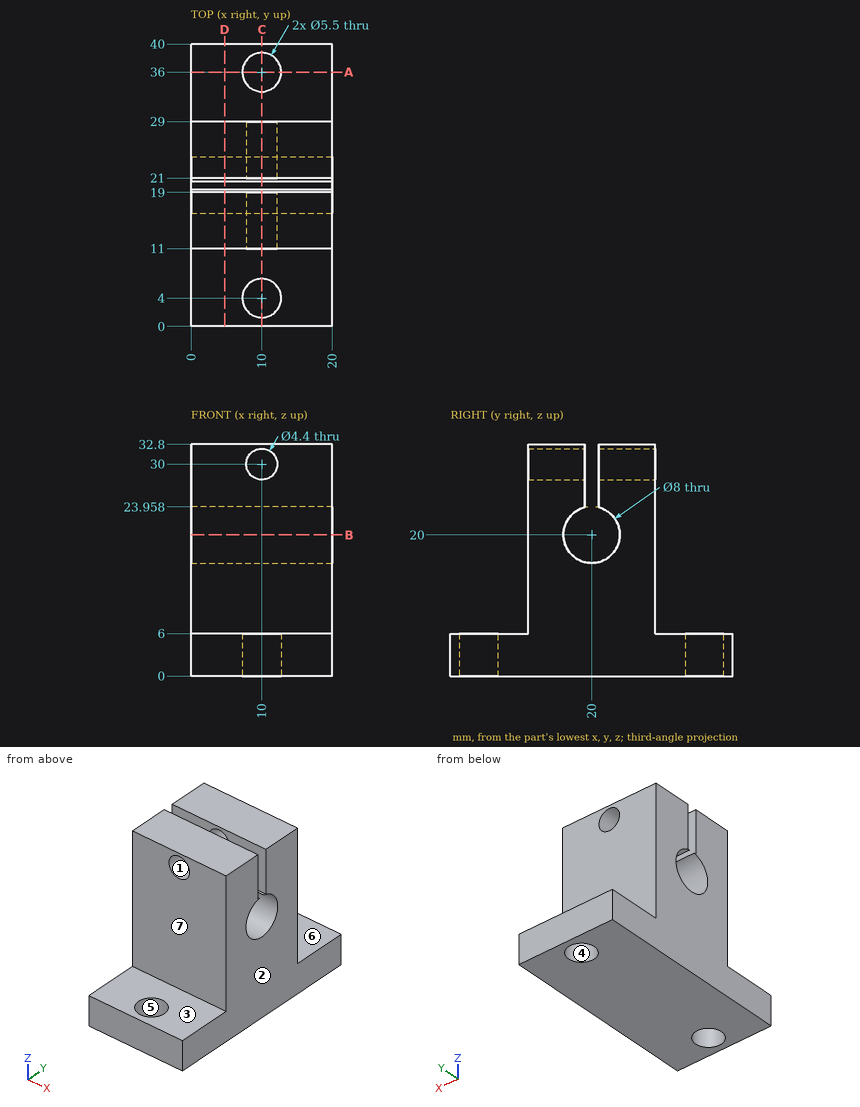
Job drawing, mm, ordinate dimensions from the low corner. One solid piece. A direction names the side the tool comes from. Round coordinates to 2 decimals unless told otherwise and drop trailing zeros. Order: outer loops, then holes, each group sorted by start corner. A loop starts at its lowest first (then second) coordinate and runs counter-clockwise, first axis right, second up. Notation, with made-up numbers: M 28.25,88 L 78.25,88 A16 cw 78.25,119 Z; hole C 44,-34.75 d5. An arc over 180 degrees is marked long. Write each question's results on one line, items separated by ' | '. Start each with the question number.
(1) Probe probe 1 along Z at (x, y) = (10, 17) (1 decimal); probe 2 along Y at (x, z) = (11, 2); probe 3 along Y at (x, z) = (2.75, 31.5). List the from-to ranges inside material, lowest first. Write a range as from..to.
(2) Saw through at D-D, the plane x = 4.75. Give the cut face in (y, z) (1 decimal).
(3) Drop flat-ended pins along their axis: pin 1 (8 mm diameter, centred on x = 16.5, z = 24.5, fed in from -Y); pin 2 (9 mm diameter, centred on x = 10, y = 4, fed in from +Z); pin 3 (8 mm diameter, centred on x = 2, z = 16.5, fed in from +Y). Give the stop position or say it passes through.
(4) Which spindle directions (+Z, -Z, +X, -X, +Y, -Y) get a long thin tool onto all of the face, cutting with end or side? Do the marked faces 5, 6 and 7. Say none if no direction does.
(5) Saw through at B-B, the plane z = 20. Give the cut face in (x, y).
(6) Saw through at C-C, the plane x = 10. State how many separate pieces and enclosed holes the cut face has, then the cut area to 3 significant figures.
(7) Two-plate mould, pull along X, no slides. Class the marked faces 1, 2, 3 and 4: pulls with the +X half, pulls with the -X half, needs draft (parallel to the pull), parting line crosses it, or undercut.
(8) Saw through at A-A, the plane y = 36. Give the cut face in (x, z).
Established:
1) probe 1: z = 0..17.4, 22.6..27.8, 32.2..32.8 | probe 2: y = 0..1.44, 6.56..33.44, 38.56..40 | probe 3: y = 11..19, 21..29
2) outline: M 0,0 L 40,0 L 40,6 L 29,6 L 29,32.8 L 21,32.8 L 21,24 L 20.6,24 A4 cw long 19.4,24 L 19,24 L 19,32.8 L 11,32.8 L 11,6 L 0,6 Z
3) pin 1: stops at y = 11 | pin 2: stops at z = 6 | pin 3: stops at y = 29
4) face 5: +Z, -Z | face 6: +Z, +X, -X, +Y | face 7: +Z, +X, -X, -Y
5) outline: M 0,11 L 20,11 L 20,16 L 0,16 Z; M 0,24 L 20,24 L 20,29 L 0,29 Z
6) separate pieces: 5 | enclosed holes: 0 | area: 518 mm^2
7) face 1: undercut | face 2: pulls with the +X half | face 3: needs draft | face 4: undercut
8) outline: M 0,0 L 7.25,0 L 7.25,6 L 0,6 Z; M 12.75,0 L 20,0 L 20,6 L 12.75,6 Z
